from build123d import *

# Parameters (mm, degrees)
SKETCH1_W                   = 224.46234
SKETCH1_H                   = 149.606
BOSS_EXTRUDE1_DEPTH         = 2.54
SKETCH2_W                   = 44.45
SKETCH2_H                   = 87.5411
CUT_EXTRUDE1_DEPTH          = 135.899132423
FILLET1_R                   = 20.0025
F_1_4_CLEARANCE_HOLE1_D     = 6.5278
F_1_4_CLEARANCE_HOLE1_DEPTH = 9.398
F_1_4_CLEARANCE_HOLE1_TIP   = 1.961148974
SKETCH6_W                   = 25.4
SKETCH6_H                   = 2.54
CUT_EXTRUDE2_DEPTH          = 135.899132423
LPATTERN1_COUNT             = 4
LPATTERN1_PITCH             = 50.8
SKETCH7_W                   = 2.54
SKETCH7_H                   = 21.59
CUT_EXTRUDE3_DEPTH          = 135.899132423
LPATTERN2_COUNT             = 3
LPATTERN2_PITCH             = 43.18
SKETCH8_R                   = 9.525
CUT_EXTRUDE4_DEPTH          = 135.899132423
SKETCH9_R                   = 15.875
SKETCH9_W                   = 44.7802
SKETCH9_H                   = 50.8
CUT_EXTRUDE5_DEPTH          = 135.899132423
FILLET2_R                   = 12.7
M3_CLEARANCE_HOLE1_D        = 3.2
M3_CLEARANCE_HOLE1_DEPTH    = 9.398
M3_CLEARANCE_HOLE1_TIP      = 0.96137699
SKETCH16_W                  = 2.54
SKETCH16_H                  = 25.4
BOSS_EXTRUDE2_DEPTH         = 2.54
LPATTERN3_COUNT             = 3
LPATTERN3_PITCH             = 50.8
SKETCH18_W                  = 2.54
SKETCH18_H                  = 5.334
CUT_EXTRUDE7_DEPTH          = 141.002899371


with BuildPart() as part:
    # Sketch1 → Boss-Extrude1 (new body)
    with BuildSketch(Plane(origin=(0, 0, 0), x_dir=(0, 0, -1), z_dir=(1, 0, 0))):
        Rectangle(SKETCH1_W, SKETCH1_H)
    extrude(amount=BOSS_EXTRUDE1_DEPTH)

    # Sketch2 → Cut-Extrude1 (cut, through all)
    with BuildSketch(Plane(origin=(2.54, 0, 0), x_dir=(0, 0, -1), z_dir=(1, 0, 0))):
        with Locations((90.00617, 31.03245)):
            Rectangle(SKETCH2_W, SKETCH2_H)
    extrude(amount=-CUT_EXTRUDE1_DEPTH, mode=Mode.SUBTRACT)

    # Fillet1
    fillet1_edges = [part.edges().sort_by_distance(p)[0] for p in [
        (1.27, -12.7381, -112.23117),
    ]]
    fillet(fillet1_edges, radius=FILLET1_R)

    # 1/4 Clearance Hole1
    with Locations(Plane(origin=(2.54, 0, 0), x_dir=(0, 0, -1), z_dir=(1, 0, 0))):
        with Locations((-81.69783, -64.77), (-62.01283, -64.77), (102.09657, -64.77), (82.41157, -64.77)):
            Hole(F_1_4_CLEARANCE_HOLE1_D / 2, depth=F_1_4_CLEARANCE_HOLE1_DEPTH)
            with Locations((0, 0, -(F_1_4_CLEARANCE_HOLE1_DEPTH + F_1_4_CLEARANCE_HOLE1_TIP / 2))):  # 118° drill point
                Cone(0, F_1_4_CLEARANCE_HOLE1_D / 2, F_1_4_CLEARANCE_HOLE1_TIP, mode=Mode.SUBTRACT)

    # Sketch6 → Cut-Extrude2 (cut, through all)
    with BuildSketch(Plane(origin=(2.54, 0, 0), x_dir=(0, 0, -1), z_dir=(1, 0, 0))):
        with Locations((39.84117, 73.533)):
            Rectangle(SKETCH6_W, SKETCH6_H)
    cut_extrude2 = extrude(amount=-CUT_EXTRUDE2_DEPTH, mode=Mode.SUBTRACT)

    # LPattern1: Cut-Extrude2 ×4
    with Locations(*[(0, 0, i * LPATTERN1_PITCH) for i in range(1, LPATTERN1_COUNT)]):
        add(cut_extrude2, mode=Mode.SUBTRACT)

    # Sketch7 → Cut-Extrude3 (cut, through all)
    with BuildSketch(Plane(origin=(2.54, 0, 0), x_dir=(0, 0, -1), z_dir=(1, 0, 0))):
        with Locations((66.51117, 53.213)):
            Rectangle(SKETCH7_W, SKETCH7_H)
    cut_extrude3 = extrude(amount=-CUT_EXTRUDE3_DEPTH, mode=Mode.SUBTRACT)

    # LPattern2: Cut-Extrude3 ×3
    with Locations(*[(0, -i * LPATTERN2_PITCH, 0) for i in range(1, LPATTERN2_COUNT)]):
        add(cut_extrude3, mode=Mode.SUBTRACT)

    # Sketch8 → Cut-Extrude4 (cut, through all)
    with BuildSketch(Plane(origin=(2.54, 0, 0), x_dir=(0, 0, -1), z_dir=(1, 0, 0))):
        with Locations((92.22867, -39.7370046)):
            Circle(SKETCH8_R)
        with Locations((-71.82993, -39.7370046)):
            Circle(SKETCH8_R)
    extrude(amount=-CUT_EXTRUDE4_DEPTH, mode=Mode.SUBTRACT)

    # Sketch9 → Cut-Extrude5 (cut, through all)
    with BuildSketch(Plane(origin=(2.54, 0, 0), x_dir=(0, 0, -1), z_dir=(1, 0, 0))):
        with Locations((-67.78625, 31.7373)):
            Circle(SKETCH9_R)
        with Locations((3.84937, -30.353)):
            Rectangle(SKETCH9_W, SKETCH9_H)
    extrude(amount=-CUT_EXTRUDE5_DEPTH, mode=Mode.SUBTRACT)

    # Fillet2
    fillet2_edges = [part.edges().sort_by_distance(p)[0] for p in [
        (1.27, -55.753, 18.54073),
        (1.27, -4.953, 18.54073),
        (1.27, -4.953, -26.23947),
        (1.27, -55.753, -26.23947),
    ]]
    fillet(fillet2_edges, radius=FILLET2_R)

    # M3 Clearance Hole1
    with Locations(Plane(origin=(2.54, 0, 0), x_dir=(0, 0, -1), z_dir=(1, 0, 0))):
        with Locations((-102.70617, 62.738), (55.71617, 62.738)):
            Hole(M3_CLEARANCE_HOLE1_D / 2, depth=M3_CLEARANCE_HOLE1_DEPTH)
            with Locations((0, 0, -(M3_CLEARANCE_HOLE1_DEPTH + M3_CLEARANCE_HOLE1_TIP / 2))):  # 118° drill point
                Cone(0, M3_CLEARANCE_HOLE1_D / 2, M3_CLEARANCE_HOLE1_TIP, mode=Mode.SUBTRACT)

    # Sketch16 → Boss-Extrude2 (add)
    with BuildSketch(Plane(origin=(2.54, 0, 0), x_dir=(0, 0, -1), z_dir=(1, 0, 0))):
        with Locations((-113.50117, 34.163)):
            Rectangle(SKETCH16_W, SKETCH16_H)
    boss_extrude2 = extrude(amount=-BOSS_EXTRUDE2_DEPTH)

    # LPattern3: Boss-Extrude2 ×3
    with Locations(*[(0, -i * LPATTERN3_PITCH, 0) for i in range(1, LPATTERN3_COUNT)]):
        add(boss_extrude2)

    # Sketch18 → Cut-Extrude7 (cut, through all)
    with BuildSketch(Plane(origin=(2.54, 0, 0), x_dir=(0, 0, -1), z_dir=(1, 0, 0))):
        with Locations((-113.50117, -77.47)):
            Rectangle(SKETCH18_W, SKETCH18_H)
    extrude(amount=-CUT_EXTRUDE7_DEPTH, mode=Mode.SUBTRACT)


solid = part.part
The listing builds one solid part. Answer for the finished solid, in the listing's coordinates (mm). A direction names the side the tool comes from. Coordinates: 2 decimals unless noted, no trailing zeros. Order: outer loops, then holes, each group sorted by start corner. A loop starts at its lowest first (then second) coordinate and runs counter-clockwise, first axis right, second up.
Q1. A cutting plane is placed at B-B, the plane y = 39. Write down the section's boundary in (x, z), and give its area (3 significant figures).
Q2. Which of the six approach directions +Z, -Z, +X, -X, +Y, -Y give full straight-line access (tool end or side, diameter ignored) to faces 5 (the face through (0, 1, 28)), 6 (the face through (1.252, -52.131, 14.722))?
Q3. A cutting plane is placed at C-C, the plane z = -96. Write down the section's boundary in (x, y), and give its area (3 significant figures).
Q4. For a pull along Z with two mould halves and no side action, classify faces 1 (the face through (2.54, 1, 28)), 2 (the face through (1.252, -18.753, -106.527)), 3 (the face through (1.288, -39.318, 81.346)), 4 (the face through (1.288, -39.318, -82.713)) as pulls with the +Z half, pulls with the -Z half, needs draft (parallel to the pull), parting line crosses it, or undercut.
Q5. Consider line 1 (Y direction, x = 0.3, z = 69); line 2 (Y direction, x = 0.85, z = -91.5); line 3 (Y direction, x = 2.25, z = -85). Determine where each line is inside the solid, lowest interval first.
Q6. A cutting plane is placed at D-D, the plane z = -37. Write down the section's boundary in (x, y).
Q7. Given P1, Ø1.3, axis at x = 2, z = 57.5, coming from the +Y side; P2, Ø1.3, axis at x = 1.5, y = 13.5, coming from the +Z side; P3, Ø0.8, axis at x = 1, y = -6, coming from the -Z side, each flat-ended and moving along its own axis, determine where each tip first touches the part or whether it passes through.
Q8. A cutting plane is placed at A-A, the plane y = -64.77. Write down the section's boundary in (x, z).
Answers follow:
1. outline: (0, -67.78) - (2.54, -67.78) - (2.54, 53.67) - (0, 53.67) - close; (0, 81.9) - (2.54, 81.9) - (2.54, 114.77) - (0, 114.77) - close
1. area: 392 mm2
2. face 5: +Z, -Z, -X, +Y, -Y
2. face 6: +X, -X
3. outline: (0, -74.8) - (2.54, -74.8) - (2.54, -48.48) - (0, -48.48) - close; (0, -30.99) - (2.54, -30.99) - (2.54, -13.1) - (0, -13.1) - close
3. area: 112 mm2
4. face 1: needs draft
4. face 2: pulls with the -Z half
4. face 3: undercut
4. face 4: undercut
5. line 1: y = -74.8 to -48.83, -30.64 to 15.91, 47.57 to 72.26
5. line 2: y = -74.8 to -49.23, -30.24 to -12.74
5. line 3: y = -74.8 to -66.76, -62.78 to -45.94, -33.53 to -12.74
6. outline: (0, -74.8) - (2.54, -74.8) - (2.54, 72.26) - (0, 72.26) - close
7. P1: stops at y = 72.26
7. P2: stops at z = 112.23
7. P3: stops at z = -67.78
8. outline: (0, -112.23) - (2.54, -112.23) - (2.54, -105.36) - (0, -105.36) - close; (0, -98.83) - (2.54, -98.83) - (2.54, -85.68) - (0, -85.68) - close; (0, -79.15) - (2.54, -79.15) - (2.54, 58.75) - (0, 58.75) - close; (0, 65.28) - (2.54, 65.28) - (2.54, 78.43) - (0, 78.43) - close; (0, 84.96) - (2.54, 84.96) - (2.54, 114.77) - (0, 114.77) - close
